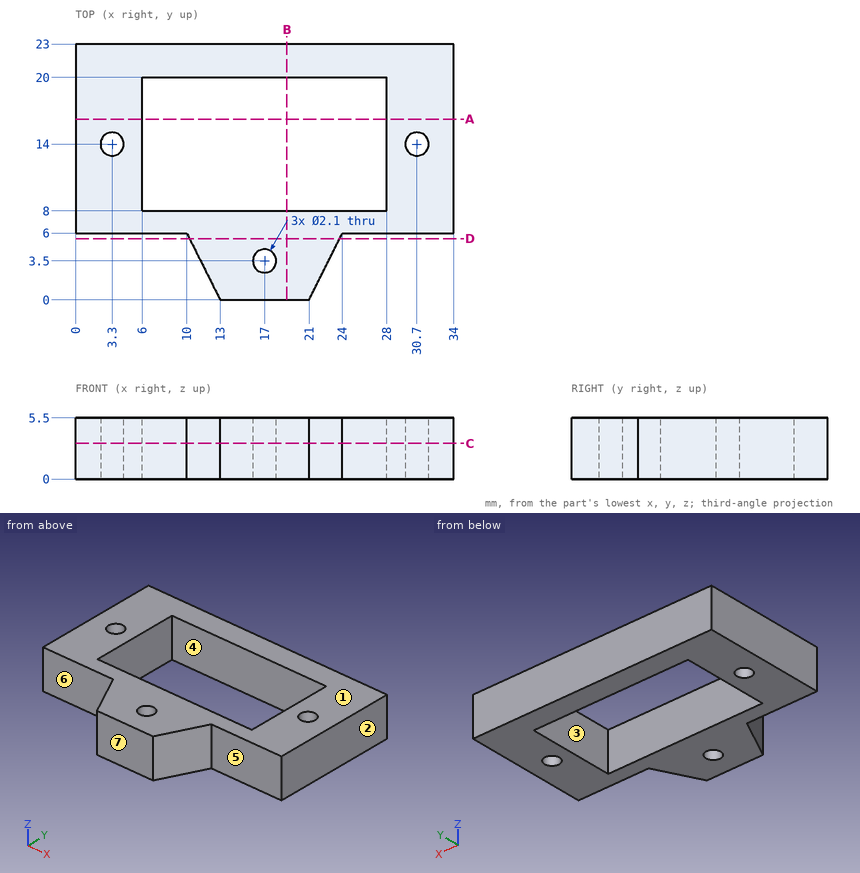
Geometry: see drawing. Coordinates: mm, zero at the bounding-box minimum. A direction names the side the tool comes from. Round coordinates to 2 decimals unless told otherwise and drop trailing zeros. Loops run counter-clockwise (first coordinate to the right, second up) from the corner with the lowest first, then second, coordinate; pieces in that order, holes last. Notation, with made-up numbers: M -30,2 L 16,2 A9 ccw 16,11 Z; hole C 74,-20.5 d8. An arc over 180 degrees is marked long. Use a Markdown table: item, result. Add a question column.
1. Section query A-A on y = 16.25. Return the cut outline in (x, z).
2. Section query C-C on z = 3.2. Return the cut outline in (x, y).
3. Section query D-D on y = 5.5. Return the cut outline in (x, z), then the cut area to 4 significant figures.
4. Reachability of the marked faces 4, 5, 6 and 7 from +Z, -Z, +X, -X, +Y, -Y: full face, straight path, thin tool, end or side. Return the list, or none.
5. Mould query, pull axis X, two halves, no side actions, for the marked faces 1, 2 and 3. Classes: pulls with the +X half, pulls with the -X half, needs draft (parallel to the pull), parting line crosses it, or undercut.
6. Contact query for flat-ended pins moving along their axis: P1, Ø1.6, axis at x = 31, z = 2.5, coming from the -Y side; P2, Ø6, axis at x = 24, y = 9, coming from the +Z side; P3, Ø2, axis at x = 11, z = 1, coming from the -Y side. Output: stop coordinate, or through.
7. Section query B-B on x = 19. Return the cut outline in (y, z).
8. Line query: line 1 (Y direction, x = 8.5, z = 1.55); line 2 (Y direction, x = 14, z = 0.6); line 3 (Y direction, x = 17, z = 1.25). Output: solid intervals per line, ascending.
Reported:
| question | item | result |
|---|---|---|
| 1 | outline | M 0,0 L 6,0 L 6,5.5 L 0,5.5 Z; M 28,0 L 34,0 L 34,5.5 L 28,5.5 Z |
| 2 | outline | M 0,6 L 10,6 L 13,0 L 21,0 L 24,6 L 34,6 L 34,23 L 0,23 Z; hole C 3.3,14 d2.1; hole M 6,8 L 28,8 L 28,20 L 6,20 Z; hole C 17,3.5 d2.1; hole C 30.7,14 d2.1 |
| 3 | outline | M 10.25,0 L 23.75,0 L 23.75,5.5 L 10.25,5.5 Z |
| 3 | area | 74.25 mm² |
| 4 | face 4 | +Z, -Z |
| 4 | face 5 | +Z, -Z, +X, -Y |
| 4 | face 6 | +Z, -Z, -X, -Y |
| 4 | face 7 | +Z, -Z, +X, -X, -Y |
| 5 | face 1 | needs draft |
| 5 | face 2 | pulls with the +X half |
| 5 | face 3 | undercut |
| 6 | P1 | stops at y = 6 |
| 6 | P2 | stops at z = 5.5 |
| 6 | P3 | stops at y = 2 |
| 7 | outline | M 0,0 L 8,0 L 8,5.5 L 0,5.5 Z; M 20,0 L 23,0 L 23,5.5 L 20,5.5 Z |
| 8 | line 1 | y = 6 to 8, 20 to 23 |
| 8 | line 2 | y = 0 to 8, 20 to 23 |
| 8 | line 3 | y = 0 to 2.45, 4.55 to 8, 20 to 23 |
